from build123d import *

# Parameters (mm, degrees)
F0_W     = 20.1616674036
F0_H     = 16.8965275351
F0_W_2   = 30.5136305556
F0_H_2   = 10.0199187398
F0_H_3   = 33.4494321883
F1_DEPTH = 76.2
F0_W_3   = 36.9883325964
F2_DEPTH = 50.8
F0_W_4   = 32.9863694444
F3_DEPTH = 38.1
F4_DEPTH = 25.4


with BuildPart() as f1:
    # F0 (on Top) → F1 (new body)
    with BuildSketch(Plane.XY):
        with Locations((-25.5707731128, 16.4976959558)):
            Rectangle(F0_W, F0_H)
        Polygon((-35.6516068146, 25.4), (-35.6516068146, 24.9459597234), (-15.489939411, 24.9459597234), (-15.489939411, 8.0494321883), (-15.3652373701, 8.0494321883), (-15.3652373701, 18.0693509281), (15.1483931854, 18.0693509281), (15.1483931854, 25.4), align=None)
        with Locations((-0.1084220923, 13.0593915582)):
            Rectangle(F0_W_2, F0_H_2)
        with Locations((-0.1084220923, -8.6752839059)):
            Rectangle(F0_W_2, F0_H_3)
        with Locations((-25.5707731128, -8.6752839059)):
            Rectangle(F0_W, F0_H_3)
    extrude(amount=F1_DEPTH)

    # F0 (on Top) → F2 (join)
    with BuildSketch(Plane.XY):
        Polygon((-72.639939411, 24.9459597234), (-85.339939411, 24.9459597234), (-85.339939411, -51.2540402766), (-15.489939411, -51.2540402766), (-15.489939411, -25.4), (-35.6516068146, -25.4), (-35.6516068146, 8.0494321883), (-72.639939411, 8.0494321883), align=None)
        with Locations((-54.1457731128, 16.4976959558)):
            Rectangle(F0_W_3, F0_H)
    extrude(amount=F2_DEPTH)

    # F0 (on Top) → F3 (join)
    with BuildSketch(Plane.XY):
        Polygon((-72.639939411, 46.1494321883), (-72.639939411, 24.9459597234), (-35.6516068146, 24.9459597234), (-35.6516068146, 25.4), (15.1483931854, 25.4), (15.1483931854, 18.0693509281), (48.1347626299, 18.0693509281), (48.1347626299, 8.0494321883), (54.360060589, 8.0494321883), (54.360060589, 46.1494321883), align=None)
        with Locations((31.6415779077, 13.0593915582)):
            Rectangle(F0_W_4, F0_H_2)
    extrude(amount=F3_DEPTH)

    # F0 (on Top) → F4 (join)
    with BuildSketch(Plane.XY):
        Polygon((15.1483931854, -25.4), (-15.3652373701, -25.4), (-15.3652373701, -45.4306490719), (48.1347626299, -45.4306490719), (48.1347626299, 8.0494321883), (15.1483931854, 8.0494321883), align=None)
    extrude(amount=F4_DEPTH)


solid = f1.part
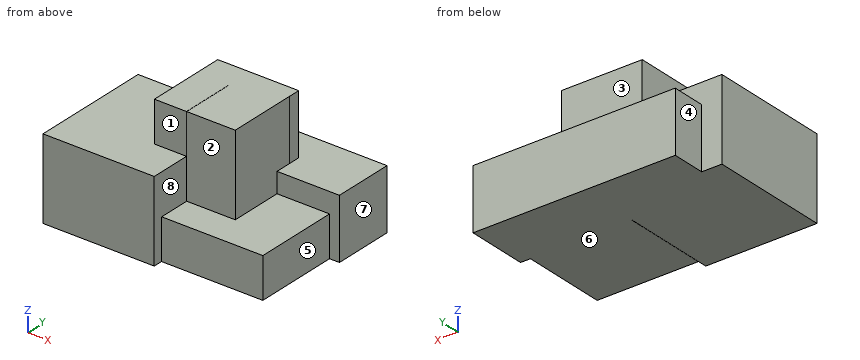
Could you check a few things on this model? Use its own coordinates, in mm. Face numbers are marked on the shaded views. A direction names the side the tool comes from. Give positions to 0.01 mm unless a question says otherwise; leave off trailing zeros. Order: outer loops, then holes, each group sorted by start corner. A loop starts at its lowest first (then second) coordinate and runs counter-clockwise, first axis right, second up. Notation, with made-up numbers: (14, -6) - (40, -6) arc R31 ccw to (40, 31) - close; hole circle Ø4 at (-32, -12). An arc over 180 degrees is marked (long way). One line per item, written item: value. Start each with the question number.
1. If I drill on probe 1 along Y at (x, z) = (18, 14); probe 2 along Y at (x, z) = (-73, 18.5); probe 3 along Z at (x, y) = (-60.5, -41.5), over which ranges is the centre line in solid material (lowest first)?
2. Imagine slicing it at D-D on y = 15. List the corners of the cut face in (x, z) for me, plus the area to 3 significant figures.
3. For P1, Ø11.5, axis at x = -12, z = 66, coming from the +Y side; P2, Ø1.5, axis at x = -25, y = 34, coming from the +Z side; P3, Ø8, axis at y = 20.5, z = 52, coming from the +X side, each with a flat end and sliding along its axis, tell me the tip position at first contact or that it passes through.
4. Imagine slicing it at A-A on y = -32. List the corners of the cut face in (x, z) for me, plus the area to 3 significant figures.
5. For the marked faces 1, 2, 3, 4 and 5, which set-ups out of +Z, -Z, +X, -X, +Y, -Y let a thin tool reach every point of the face, with its end or its side?
6. Imagine slicing it at B-B on z = 63. List the corners of the cut face in (x, y) for me, plus the area to 3 significant figures.
7. Imagine slicing it at C-C on x = -56.5. List the corners of the cut face in (y, z) for me, plus the area to 3 significant figures.
8. Thinking about a two-plate mould opening in X: for the marked faces 6, 7 and 8, which applies, +X half, -X half, draft (parallel to the pull), parting line (faces both ways), or undercut?
Values:
1. probe 1: -45.43 to 46.15
1. probe 2: -51.25 to 24.95
1. probe 3: 0 to 50.8
2. outline: (-85.34, 0) - (54.36, 0) - (54.36, 38.1) - (15.15, 38.1) - (15.15, 76.2) - (-35.65, 76.2) - (-35.65, 50.8) - (-85.34, 50.8) - close
2. area: 7,890 mm²
3. P1: y = 25.4
3. P2: z = 38.1
3. P3: x = 15.15
4. outline: (-85.34, 0) - (-15.49, 0) - (-15.49, 50.8) - (-85.34, 50.8) - close; (-15.37, 0) - (48.13, 0) - (48.13, 25.4) - (-15.37, 25.4) - close
4. area: 5,160 mm²
5. face 1: +Z, +X, -X, -Y
5. face 2: +Z, +X, -Y
5. face 3: +Z, +X, -X, +Y
5. face 4: +Z, -Z, -X, +Y
5. face 5: +Z, -Z, +X, -Y
6. outline: (-35.65, -25.4) - (-15.49, -25.4) - (-15.49, 8.05) - (-15.37, 8.05) - (-15.37, -25.4) - (15.15, -25.4) - (15.15, 25.4) - (-35.65, 25.4) - close
6. area: 2,580 mm²
7. outline: (-51.25, 0) - (46.15, 0) - (46.15, 38.1) - (24.95, 38.1) - (24.95, 50.8) - (-51.25, 50.8) - close
7. area: 4,680 mm²
8. face 6: draft
8. face 7: +X half
8. face 8: undercut
